Model file for the job. Use its own axes, mm. A direction names the side the tool comes from. Coordinates: 2 decimals unless noted, no trailing zeros. Order: outer loops, then holes, each group sorted by start corner. A loop starts at its lowest first (then second) coordinate and runs counter-clockwise, first axis right, second up. Notation, with made-up numbers: (74.25, 63.5) -> (114.25, 63.5) arc R25 cw to (114.25, 84.5) -> close; hole circle Ø6 at (34.25, -16.75). An arc over 180 degrees is marked (long way). Return JSON: item names as keys, results as strings. Group by question number.
1) Probe line 1 (Y direction, x = -3, z = -5); line 2 (Z direction, x = 0, y = 1.2); line 3 (X direction, y = 21.5, z = 13.75). List the from-to ranges inside material, lowest first.
2) Cut at B-B (y = 35). Write the cut outline in (x, z).
3) Pull direction X, two halves, no side cores. Call faces 6 (the cylindrical face through (6, 35, 0)), 7 (the flat face through (0, 37, 0)), 8 (the cylindrical face through (0, 39, -4)): +X half, -X half, draft (parallel to the pull), parting line (faces both ways), or undercut.
4) Cut at D-D (x = 0). State how many separate pieces and enclosed holes the cut face has, and give its area (3 significant figures).
5) Cut at C-C (x = -11.5). Write the cut outline in (y, z), and give its area (3 significant figures).
6) Flat gauge pins, fed straight in: pin 1 (3 mm diameter, centred on x = -9.5, z = -6, fed in from -Y); pin 2 (6 mm diameter, centred on x = 5.5, y = 30, fed in from -Z); pin 3 (6 mm diameter, centred on y = 22.5, z = -4, fed in from -X). Where does each tip first touch, or does it go through?
7) Cut at A-A (z = 0). Write the cut outline in (x, y).
8) Which spindle directions (+Z, -Z, +X, -X, +Y, -Y) get a long thin tool onto all of the face, cutting with end or side? Do faces 1 (the cylindrical face through (-6.466, 6.084, 2.681)), 2 (the cylindrical face through (0.1, 38.5, 5)), 3 (the cylindrical face through (-0.1, 38.5, -5)), 4 (the flat face through (-3, 12, 3)), 5 (the flat face through (1, 39, 2.5)). Say none if no direction does.
from build123d import *

# Parameters (mm, degrees)
FILLET1_R               = 3
SKETCH3_W               = 5
SKETCH3_H               = 6
CUT_EXTRUDE1_DEPTH      = 10
CUT_EXTRUDE1_DEPTH_BACK = 10
SKETCH4_R               = 1
CUT_EXTRUDE2_DEPTH      = 10
CUT_EXTRUDE2_DEPTH_BACK = 10


with BuildPart() as part:
    # Sketch2 → Revolve1 (revolve)
    with BuildSketch(Plane.XY):
        Polygon((-4, 12), (-4, 15), (-15, 15), (-15, 33), (-6, 33), (-6, 37), (-5, 37), (-5, 43), (0, 43), (0, 37), (0, 4), (-1, 4), (-1, 0), (-7, 0), (-7, 12), align=None)
    revolve(axis=Axis((0, 37, 0), (0, -1, 0)))

    # Fillet1
    fillet1_edges = [part.edges().sort_by_distance(p)[0] for p in [
        (5, 43, 0),
    ]]
    fillet(fillet1_edges, radius=FILLET1_R)

    # Sketch3 → Cut-Extrude1 (cut, two sides)
    with BuildSketch(Plane(origin=(0, 0, 0), x_dir=(0, 0, -1), z_dir=(1, 0, 0))) as cut_extrude1_sk:
        with Locations((0, 40)):
            Rectangle(SKETCH3_W, SKETCH3_H)
    extrude(amount=CUT_EXTRUDE1_DEPTH, mode=Mode.SUBTRACT)
    extrude(cut_extrude1_sk.sketch, amount=-CUT_EXTRUDE1_DEPTH_BACK, mode=Mode.SUBTRACT)

    # Sketch4 → Cut-Extrude2 (cut, two sides)
    with BuildSketch(Plane(origin=(0, 0, 2.5), x_dir=(-1, 0, 0), z_dir=(0, 0, -1))) as cut_extrude2_sk:
        with Locations((0, 40)):
            Circle(SKETCH4_R)
    extrude(amount=CUT_EXTRUDE2_DEPTH, mode=Mode.SUBTRACT)
    extrude(cut_extrude2_sk.sketch, amount=-CUT_EXTRUDE2_DEPTH_BACK, mode=Mode.SUBTRACT)


solid = part.part
Answers below:
{
 "1": {"line 1": "y = 0 to 12, 15 to 37", "line 2": "z = -7 to -1, 1 to 7", "line 3": "x = -5.99 to 5.99"},
 "2": {"outline": "circle Ø12 at (0, 0)"},
 "3": {"face 6": "parting line", "face 7": "draft", "face 8": "undercut"},
 "4": {"separate pieces": "3", "enclosed holes": "0", "area": "788 mm^2"},
 "5": {"outline": "(15, -9.63) -> (33, -9.63) -> (33, 9.63) -> (15, 9.63) -> close", "area": "347 mm^2"},
 "6": {"pin 1": "stops at y = 15", "pin 2": "stops at z = -14.79", "pin 3": "stops at x = -14.97"},
 "7": {"outline": "(-15, 15) -> (-4, 15) -> (-4, 12) -> (-7, 12) -> (-7, 0) -> (-1, 0) -> (-1, 4) -> (1, 4) -> (1, 0) -> (7, 0) -> (7, 12) -> (4, 12) -> (4, 15) -> (15, 15) -> (15, 33) -> (6, 33) -> (6, 37) -> (-6, 37) -> (-6, 33) -> (-15, 33) -> close"},
 "8": {"face 1": "-Y", "face 2": "+Z, +Y", "face 3": "-Z, +Y", "face 4": "none", "face 5": "+X, -X, +Y"}
}
